from build123d import *

# Parameters (mm, degrees)
CROQUIS1_R              = 9.525
SALIENTE_EXTRUIR1_DEPTH = 71.6
CROQUIS2_R              = 4.7625
SALIENTE_EXTRUIR2_DEPTH = 19.86
SALIENTE_EXTRUIR3_START = 19.86
CROQUIS3_R              = 4.7625
SALIENTE_EXTRUIR3_DEPTH = 19.86
CROQUIS4_R              = 2
CORTAR_EXTRUIR1_DEPTH   = 5
CORTAR_EXTRUIR2_START   = -5
CROQUIS5_R              = 2
CORTAR_EXTRUIR2_DEPTH   = 5


with BuildPart() as part:
    # Croquis1 → Saliente-Extruir1 (new body)
    with BuildSketch(Plane.XY):
        with Locations(Location((0, 0, 0), (0, 0, 180))):
            Circle(CROQUIS1_R)
    extrude(amount=SALIENTE_EXTRUIR1_DEPTH)

    # Croquis2 → Saliente-Extruir2 (add)
    with BuildSketch(Plane.XY.offset(71.6)):
        Circle(CROQUIS2_R)
    extrude(amount=SALIENTE_EXTRUIR2_DEPTH)

    # Croquis3 → Saliente-Extruir3 (add)
    with BuildSketch(Plane(origin=(0, 0, 0), x_dir=(-1, 0, 0), z_dir=(0, 0, -1)).offset(SALIENTE_EXTRUIR3_START)):
        with Locations(Location((0, 0, 0), (0, 0, 180))):
            Circle(CROQUIS3_R)
    extrude(amount=-SALIENTE_EXTRUIR3_DEPTH)

    # Croquis4 → Cortar-Extruir1 (cut)
    with BuildSketch(Plane(origin=(0, 0, -19.86), x_dir=(-1, 0, 0), z_dir=(0, 0, -1))):
        Circle(CROQUIS4_R)
    extrude(amount=-CORTAR_EXTRUIR1_DEPTH, mode=Mode.SUBTRACT)

    # Croquis5 → Cortar-Extruir2 (cut)
    with BuildSketch(Plane.XY.offset(91.46).offset(CORTAR_EXTRUIR2_START)):
        with Locations(Location((0, 0, 0), (0, 0, 180))):
            Circle(CROQUIS5_R)
    extrude(amount=CORTAR_EXTRUIR2_DEPTH, mode=Mode.SUBTRACT)


solid = part.part
Part model, mm, in its own coordinate system. A direction names the side the tool comes from. Round coordinates to 2 decimals unless told otherwise and drop trailing zeros. Write each loop counter-clockwise with the first axis right and the second up, starting at its lowest first coordinate (ties: lowest second). Pieces come first, ordered by that corner, then holes. Notation, with made-up numbers: (70, 74) - (120, 74) arc R9 cw to (120, 85) - close; hole circle Ø9 at (-2, 0). An arc over 180 degrees is marked (long way). Use CSV: the item, a comma, the result in double quotes.
Item 1: Wall check: L1, parallel to Y at x = 0, z = -16.1; L2, parallel to Z at x = -0.5, y = -0.5; L3, parallel to Z at x = -1.25, y = -7.5. Give the ranges that are in metal, low to high.
Results list:
L1,"y = -4.76 to -2, 2 to 4.76"
L2,"z = -14.86 to 86.46"
L3,"z = 0 to 71.6"
Item 2: Slice it at A-A, the plane x = 0. Write the cut outline in (y, z) (1 decimal), then the cut area to 3 significant figures.
Results list:
outline,"(-9.5, 0) - (-4.8, 0) - (-4.8, -19.9) - (-2, -19.9) - (-2, -14.9) - (2, -14.9) - (2, -19.9) - (4.8, -19.9) - (4.8, 0) - (9.5, 0) - (9.5, 71.6) - (4.8, 71.6) - (4.8, 91.5) - (2, 91.5) - (2, 86.5) - (-2, 86.5) - (-2, 91.5) - (-4.8, 91.5) - (-4.8, 71.6) - (-9.5, 71.6) - close"
area,"1,700 mm²"
Item 3: Slice it at C-C, the plane z = 55. Write the cut outline in (x, y) (3 decimals).
Results list:
outline,"circle Ø19.05 at (0, 0)"
Item 4: Tool access for faces 4 (the flat face through (2, 1, -19.86)), 5 (the cylindrical face through (0, -2, -17)), 6 (the flat face through (2.3, -4.4, 71.6)): list every direction of +Z, -Z, +X, -X, +Y, -Y with a clear straight run to the whole face (end or side of a thin tool).
Results list:
face 4,"-Z, +X, -X, +Y, -Y"
face 5,"-Z"
face 6,"+Z"
Item 5: Slice it at D-D, the plane z = 78.5. Write the cut outline in (x, y) (1 decimal), then the cut area to 3 significant figures.
Results list:
outline,"circle Ø9.5 at (0, 0)"
area,"71.3 mm²"
Item 6: Pull direction X, two halves, no side cores. Call faces 1 (the cylindrical face through (2.06, 9.3, 35.3)), 2 (the flat face through (0, 0, 86.46)), 3 (the flat face through (2, -1, 91.46)): pulls with the +X half, pulls with the -X half, needs draft (parallel to the pull), parting line crosses it, or undercut.
Results list:
face 1,"parting line crosses it"
face 2,"undercut"
face 3,"needs draft"
Item 7: Flat gauge pins, fed straight in: P1, Ø1.2, axis at x = 0, y = -0.5, coming from the -Z side; P2, Ø6, axis at x = 6, z = 0.5, coming from the +Y side; P3, Ø4, axis at y = 6.5, z = 48, coming from the +X side (3 decimals). Where does each tip first touch, or does it go through?
Results list:
P1,"stops at z = -14.86"
P2,"stops at y = 9.04"
P3,"stops at x = 8.395"
